from build123d import *

# Parameters (mm, degrees)
BOSS_EXTRUDE1_DEPTH     = 11.1125
SKETCH3_W               = 22.225
SKETCH3_H               = 22.225
BOSS_EXTRUDE2_DEPTH     = 76.2
BOSS_EXTRUDE3_DEPTH     = 22.225
SKETCH6_R               = 2.413
CUT_EXTRUDE1_DEPTH      = 83.55
CUT_EXTRUDE2_DEPTH      = 1
CUT_EXTRUDE2_DEPTH_BACK = 23.225
FILLET1_R               = 3.175
SKETCH8_R               = 3.175
CUT_EXTRUDE3_DEPTH      = 9.525


with BuildPart() as part:
    # Sketch1 → Boss-Extrude1 (new body, symmetric)
    with BuildSketch(Plane(origin=(0, 0, 0), x_dir=(0, 0, -1), z_dir=(1, 0, 0))):
        Polygon((-22.225, 6.35), (0, 6.35), (46.99, 6.35), (46.99, -3.81), (40.64, -3.81), (40.64, 0), (0, 0), (-22.225, 0), align=None)
    extrude(amount=BOSS_EXTRUDE1_DEPTH, both=True)

    # Sketch3 → Boss-Extrude2 (add)
    with BuildSketch(Plane.XZ):
        with Locations((0, 11.1125)):
            Rectangle(SKETCH3_W, SKETCH3_H)
    extrude(amount=BOSS_EXTRUDE2_DEPTH)

    # Sketch5 → Boss-Extrude3 (add)
    with BuildSketch(Plane(origin=(11.1125, 0, 0), x_dir=(0, 0, -1), z_dir=(1, 0, 0))):
        Polygon((-22.225, 6.35), (-105.41, -76.2), (-22.225, -76.2), align=None)
    extrude(amount=-BOSS_EXTRUDE3_DEPTH)

    # Sketch6 → Cut-Extrude1 (cut, through all)
    with BuildSketch(Plane.XZ.offset(76.2)):
        with Locations((0, 92.71)):
            Circle(SKETCH6_R)
        with Locations((0, 12.7)):
            Circle(SKETCH6_R)
        with Locations((0, 52.705)):
            Circle(SKETCH6_R)
    extrude(amount=-CUT_EXTRUDE1_DEPTH, mode=Mode.SUBTRACT)

    # Sketch7 → Cut-Extrude2 (cut, two sides)
    with BuildSketch(Plane.ZY.offset(11.1125)) as cut_extrude2_sk:
        Polygon((46.355, -17.595801527), (46.355, -30.198854962), (59.055, -30.198854962), align=None)
        Polygon((86.36, -57.295419847), (86.36, -69.898473282), (99.06, -69.898473282), align=None)
    extrude(amount=CUT_EXTRUDE2_DEPTH, mode=Mode.SUBTRACT)
    extrude(cut_extrude2_sk.sketch, amount=-CUT_EXTRUDE2_DEPTH_BACK, mode=Mode.SUBTRACT)

    # Fillet1
    fillet1_edges = [part.edges().sort_by_distance(p)[0] for p in [
        (0, 6.35, -46.99),
        (0, -3.81, -46.99),
    ]]
    fillet(fillet1_edges, radius=FILLET1_R)

    # Sketch8 → Cut-Extrude3 (cut)
    with BuildSketch(Plane(origin=(0, 0, 0), x_dir=(-1, 0, 0), z_dir=(0, 0, -1))):
        with Locations((0, -52.3875)):
            Circle(SKETCH8_R)
    extrude(amount=-CUT_EXTRUDE3_DEPTH, mode=Mode.SUBTRACT)


solid = part.part
Check sheet for the modelled part. Datum: model origin and axes. Units: mm. A direction names the side the tool comes from. Round coordinates to 2 decimals unless told otherwise and drop trailing zeros. Loops run counter-clockwise (first coordinate to the right, second up) from the corner with the lowest first, then second, coordinate; pieces in that order, holes last. Notation, with made-up numbers: (40.25, -21) -> (82.25, -21) arc R27 cw to (82.25, 13) -> close; hole circle Ø10 at (-10, 47.25). An arc over 180 degrees is marked (long way). Put each result on its own line as item: value. Start each with the question number.
1. Scan lines: probe 1 along Z at (x, y) = (0, -61); probe 2 along Y at (x, z) = (0, 7); probe 3 along Z at (x, y) = (2, -60.5). Record each from-to range of solid material in increasing order.
2. Draft check along X on faces 4 (the face through (-0.314, -73.093, 95.102)), 5 (the face through (-11.112, -44, 30)), 6 (the face through (-0.16, -2.86, -46.08)). Enter one of: +X half, -X half, draft (parallel to the pull), parting line (faces both ways), or undercut.
3. Section check A-A (x = 0). Give the number of separate pieces and of enclosed holes in the cut face, plus the area to 3 significant figures.
4. Section check D-D (x = -6.5). Enter the section's corners in (y, z) (3 decimals), plus the area to 3 significant figures.
5. Gauge pin test, flat ends, axial feed: pin 1 (10 mm diameter, centred on x = 4, y = -6.5, fed in from -Z); pin 2 (12 mm diameter, centred on y = -14, z = 43.5, fed in from +X); pin 3 (6.5 mm diameter, centred on x = 2.5, y = -52.5, fed in from -Z); pin 4 (6 mm diameter, centred on x = 4.5, y = -60, fed in from +Z). Record the tip position at first contact, or that the pin passes through.
6. Section check C-C (y = -28). Enter the section's corners in (x, z) (1 decimal).
7. Access from +Z, -Z, +X, -X, +Y, -Y to the whole of each face (thin tool, end or side, straight path). Record for faces 1 (the face through (-3, -30.199, 53)), 2 (the face through (0, -3.81, -42)), 3 (the face through (0, -2, -40.64)).
8. Section check B-B (z = 12.7). Enter the section's corners in (x, y).
Findings:
1. probe 1: z = 0 to 10.29, 15.11 to 50.29, 55.12 to 86.36
1. probe 2: y = -76.2 to -55.56, -49.21 to 6.35
1. probe 3: z = 0 to 11.35, 14.05 to 51.35, 54.06 to 86.36
2. face 4: undercut
2. face 5: -X half
2. face 6: draft
3. separate pieces: 4
3. enclosed holes: 0
3. area: 4,720 mm^2
4. outline: (-76.2, 0) -> (0, 0) -> (0, -40.64) -> (-3.81, -40.64) -> (-3.81, -43.815) arc R3.175 ccw to (-0.635, -46.99) -> (3.175, -46.99) arc R3.175 ccw to (6.35, -43.815) -> (6.35, 22.225) -> (-17.596, 46.355) -> (-30.199, 46.355) -> (-30.199, 59.055) -> (-57.295, 86.36) -> (-69.898, 86.36) -> (-69.898, 99.06) -> (-76.2, 105.41) -> close
4. area: 5,430 mm^2
5. pin 1: stops at z = -46.87
5. pin 2: stops at x = 11.11
5. pin 3: stops at z = 0
5. pin 4: stops at z = 86.36
6. outline: (-11.1, 0) -> (11.1, 0) -> (11.1, 46.4) -> (-11.1, 46.4) -> close; hole circle Ø4.8 at (0, 12.7)
7. face 1: +Z, +X, -X, +Y
7. face 2: -Z, +X, -X, -Y
7. face 3: +X, -X, -Y
8. outline: (-11.11, -76.2) -> (-2.41, -76.2) -> (-2.41, 6.35) -> (-11.11, 6.35) -> close; (2.41, -76.2) -> (11.11, -76.2) -> (11.11, 6.35) -> (2.41, 6.35) -> close
